from build123d import *

# Parameters (mm, degrees)
SKETCH1_W           = 145
SKETCH1_H           = 90
BOSS_EXTRUDE1_DEPTH = 5
SKETCH3_W           = 120
SKETCH3_H           = 34.25
CUT_EXTRUDE1_DEPTH  = 5
SKETCH4_W           = 5
SKETCH4_H           = 40.8
SKETCH4_H_2         = 23.1
CUT_EXTRUDE2_DEPTH  = 5
SKETCH7_W           = 50.2
SKETCH7_H           = 5
CUT_EXTRUDE3_DEPTH  = 5


with BuildPart() as part:
    # Sketch1 → Boss-Extrude1 (new body)
    with BuildSketch(Plane(origin=(0, 0, 0), x_dir=(1, 0, 0), z_dir=(0, 1, 0))):
        Rectangle(SKETCH1_W, SKETCH1_H)
    extrude(amount=BOSS_EXTRUDE1_DEPTH)

    # Sketch3 → Cut-Extrude1 (cut)
    with BuildSketch(Plane(origin=(0, 5, 0), x_dir=(1, 0, 0), z_dir=(0, 1, 0))):
        with Locations((0, -7.365)):
            Rectangle(SKETCH3_W, SKETCH3_H)
    extrude(amount=-CUT_EXTRUDE1_DEPTH, mode=Mode.SUBTRACT)

    # Sketch4 → Cut-Extrude2 (cut)
    with BuildSketch(Plane(origin=(0, 5, 0), x_dir=(1, 0, 0), z_dir=(0, 1, 0))):
        with Locations((-70, 24.6)):
            Rectangle(SKETCH4_W, SKETCH4_H)
        with Locations((-70, -33.45)):
            Rectangle(SKETCH4_W, SKETCH4_H_2)
        with Locations((70, -33.45)):
            Rectangle(SKETCH4_W, SKETCH4_H_2)
        with Locations((70, 24.6)):
            Rectangle(SKETCH4_W, SKETCH4_H)
    extrude(amount=-CUT_EXTRUDE2_DEPTH, mode=Mode.SUBTRACT)

    # Sketch7 → Cut-Extrude3 (cut)
    with BuildSketch(Plane(origin=(0, 5, 0), x_dir=(1, 0, 0), z_dir=(0, 1, 0))):
        with Locations((0, -42.5)):
            Rectangle(SKETCH7_W, SKETCH7_H)
    extrude(amount=-CUT_EXTRUDE3_DEPTH, mode=Mode.SUBTRACT)


solid = part.part
Here's how the part is built. I have some questions about the finished solid (model axes, mm). A direction names the side the tool comes from. Round coordinates to 2 decimals unless told otherwise and drop trailing zeros. Loops run counter-clockwise (first coordinate to the right, second up) from the corner with the lowest first, then second, coordinate; pieces in that order, holes last.
1. For P1, Ø2.5, axis at y = 2.5, z = -19, coming from the +X side; P2, Ø2.5, axis at x = -70, y = 2.5, coming from the +Z side; P3, Ø1.5, axis at x = 16, y = 1.5, coming from the +Z side, each with a flat end and sliding along its axis, tell me the tip position at first contact or that it passes through.
Answer list:
P1: stops at x = 67.5
P2: stops at z = 21.9
P3: stops at z = 40
2. We'd pull the mould along X, two halves only. Please class faces 1 (the face through (67.5, 3, -24)), 2 (the face through (46, 2, 45)), 3 (the face through (-1, 3, -9.76)), 4 (the face through (-60, 3, 8)): +X half, -X half, draft (parallel to the pull), parting line (faces both ways), or undercut.
Answer list:
face 1: +X half
face 2: draft
face 3: undercut
face 4: undercut
3. If we section it at D-D on z = -31.5: Write out the boundary of the cut face in (x, y), plus the area to 3 significant figures.
Answer list:
outline: (-67.5, 0) - (67.5, 0) - (67.5, 5) - (-67.5, 5) - close
area: 675 mm2
4. Which directions (+Z, -Z, +X, -X, +Y, -Y) give clear straight access to the entire face, cutting with the end or side of a thin tool? Please do faces 5 (the face through (25.1, 3, 43)), 6 (the face through (-67.5, 3, 34)), 7 (the face through (60, 3, 8)), 8 (the face through (70, 3, -4.2)), 9 (the face through (67.5, 3, 34)).
Answer list:
face 5: +Z, +Y, -Y
face 6: +Z, -X, +Y, -Y
face 7: +Y, -Y
face 8: -Z, +X, +Y, -Y
face 9: +Z, +X, +Y, -Y
5. If we section it at B-B on z = 1: Write out the boundary of the cut face in (x, y).
Answer list:
outline: (-72.5, 0) - (-60, 0) - (-60, 5) - (-72.5, 5) - close; (60, 0) - (72.5, 0) - (72.5, 5) - (60, 5) - close
6. If we section it at A-A on x = 55: Write out the boundary of the cut face in (y, z).
Answer list:
outline: (0, -45) - (5, -45) - (5, -9.76) - (0, -9.76) - close; (0, 24.49) - (5, 24.49) - (5, 45) - (0, 45) - close
7. If I drill on line 1 along Z through (x, y) = (-55.5, 3); line 2 along Z through (x, y) = (-25, 0.5); line 3 along X through (y, z) = (1.25, 11), over which ranges is the centre line in solid material (lowest first)?
Answer list:
line 1: z = -45 to -9.76, 24.49 to 45
line 2: z = -45 to -9.76, 24.49 to 40
line 3: x = -72.5 to -60, 60 to 72.5
8. If we section it at C-C on y = 0.9: Write out the boundary of the cut face in (x, z), plus the area to 3 significant figures.
Answer list:
outline: (-72.5, -4.2) - (-67.5, -4.2) - (-67.5, -45) - (67.5, -45) - (67.5, -4.2) - (72.5, -4.2) - (72.5, 21.9) - (67.5, 21.9) - (67.5, 45) - (25.1, 45) - (25.1, 40) - (-25.1, 40) - (-25.1, 45) - (-67.5, 45) - (-67.5, 21.9) - (-72.5, 21.9) - close; hole (-60, -9.76) - (60, -9.76) - (60, 24.49) - (-60, 24.49) - close
area: 8,050 mm2
